Source: CAD feature listing. Evaluate the final solid. Frame: model axes, mm. Face numbers are marked on the shaded views. A direction names the side the tool comes from. Coordinates: 2 decimals unless noted, no trailing zeros. Write each loop counter-clockwise with the first axis right and the second up, starting at its lowest first coordinate (ties: lowest second). Pieces come first, ordered by that corner, then holes. Notation, with made-up numbers: M 65.25,-33 L 92.25,-33 A26 ccw 92.25,4 Z; hole C -7.5,72 d1. An arc over 180 degrees is marked long. One line per item, written item: value. Start each with the question number.
Item 1: Cut plane B-B, the plane x = 7.25. Output: boundary loops of the cut face in (y, z), then the cut area to 3 significant figures.
Item 2: Pin query (flat end, axial travel): P1, Ø3, axis at x = 1, z = 21.5, coming from the +Y side; P2, Ø8.5, axis at x = 3, z = 20.5, coming from the +Y side; P3, Ø7.5, axis at y = 19.5, z = 31, coming from the -X side. Return the tip coordinate at first contact, or that it passes through.
Item 3: Set-up query: the marked faces 1, 2, 3, 4 and 5. Return all of +Z, -Z, +X, -X, +Y, -Y with unobstructed straight access to the full face (end or side cutting, diameter ignored); none if empty.
Item 4: Cut plane C-C, the plane y = 19.5. Output: boundary loops of the cut face in (x, z), then the cut area to 3 significant figures.
Item 5: Cut plane A-A, the plane z = 8. Output: boundary loops of the cut face in (x, y).
Item 6: Ray query, L1, parallel to Y at x = -3, z = 7.5; L2, parallel to X at y = 21, z = 29.5; L3, parallel to X at y = -7, z = 20. Return the intervals inside material, ascending. Write a range as from..to.
Item 7: Cut plane D-D, the plane z = 29.5. Output: boundary loops of the cut face in (x, y).
```python
from build123d import *

# Parameters (mm, degrees)
SKETCH_1_W      = 23
SKETCH_1_H      = 19
EXTRUDE_1_DEPTH = 34
SKETCH_2_W      = 10
SKETCH_2_H      = 7
EXTRUDE_2_DEPTH = 25
FILLET_1_R      = 3


with BuildPart() as part:
    # Sketch 1 → Extrude 1 (new body)
    with BuildSketch(Plane.XY):
        Rectangle(SKETCH_1_W, SKETCH_1_H)
    extrude(amount=EXTRUDE_1_DEPTH)

    # Sketch 2 → Extrude 2 (add)
    with BuildSketch(Plane(origin=(0, 9.5, 0), x_dir=(1, 0, 0), z_dir=(0, 1, 0))):
        with Locations((0, -30.5)):
            Rectangle(SKETCH_2_W, SKETCH_2_H)
    extrude(amount=EXTRUDE_2_DEPTH)

    # Fillet 1
    fillet_1_edges = [part.edges().sort_by_distance(p)[0] for p in [
        (-5, 9.5, 30.5),
        (5, 9.5, 30.5),
        (0, 9.5, 27),
        (-5, 34.5, 30.5),
        (5, 34.5, 30.5),
        (11.5, -9.5, 17),
        (-11.5, -9.5, 17),
        (-11.5, 9.5, 17),
        (11.5, 9.5, 17),
    ]]
    fillet(fillet_1_edges, radius=FILLET_1_R)


solid = part.part
```
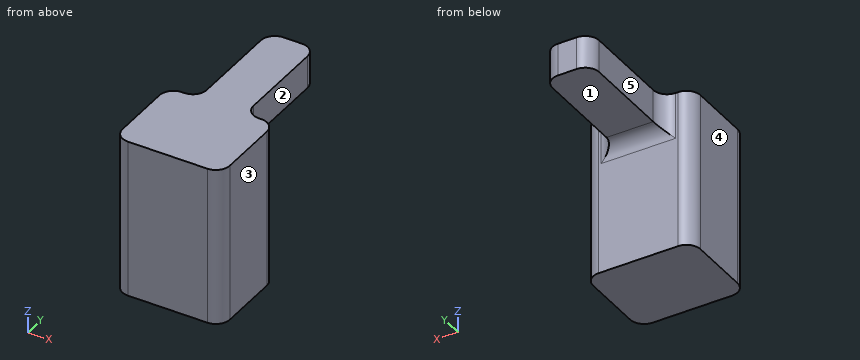
From the geometry:
1. outline: M -9.5,0 L 9.5,0 L 9.5,24 A3 cw 9.6,24.75 L 9.6,34 L -9.5,34 Z
1. area: 647 mm²
2. P1: stops at y = 9.5
2. P2: stops at y = 9.6
2. P3: stops at x = -5
3. face 1: -Z, +X, -X, +Y
3. face 2: +Z, -Z, +X, +Y
3. face 3: +Z, -Z, +X, +Y, -Y
3. face 4: +Z, -Z, -X, +Y, -Y
3. face 5: +Z, -Z, -X, +Y
4. outline: M -5,27 L 5,27 L 5,34 L -5,34 Z
4. area: 70.0 mm²
5. outline: M -11.5,-6.5 A3 ccw -8.5,-9.5 L 8.5,-9.5 A3 ccw 11.5,-6.5 L 11.5,6.5 A3 ccw 8.5,9.5 L -8.5,9.5 A3 ccw -11.5,6.5 Z
6. L1: y = -9.5..9.5
6. L2: x = -5..5
6. L3: x = -11.46..11.46
7. outline: M -11.5,-6.5 A3 ccw -8.5,-9.5 L 8.5,-9.5 A3 ccw 11.5,-6.5 L 11.5,6.5 A3 ccw 8.5,9.5 L 8,9.5 A3 cw 5,12.5 L 5,31.5 A3 ccw 2,34.5 L -2,34.5 A3 ccw -5,31.5 L -5,12.5 A3 cw -8,9.5 L -8.5,9.5 A3 ccw -11.5,6.5 Z
